Part print with two shaded views. Sizes in mm from the minimum x, y, z corner. Round coordinates to 2 decimals unless told otherwise and drop trailing zeros. Loops run counter-clockwise (first coordinate to the right, second up) from the corner with the lowest first, then second, coordinate; pieces in that order, holes last.
(1) Cut at A-A on z = 0.8. List the corners of the cut face in (x, y) (1 decimal).
(2) Cut at B-B on x = 2. List the corners of the cut face in (y, z).
(3) Cut at D-D on y = 14.5. List the corners of the cut face in (x, z).
(4) Flat gauge pin, fed straight in: pin 1 (5 mm diameter, centred on x = 8, y = 10, fed in from +Z). Where does the tip first touch, or does it go through?
(5) Probe probe 1 along Y at (x, z) = (15, 0.1); probe 2 along Y at (x, z) = (2, 0.3); probe 3 along Z at (x, y) = (1.25, 25.25). List the from-to ranges inside material, lowest first.
(6) Cut at C-C on y = 25. List the corners of the cut face in (x, z).
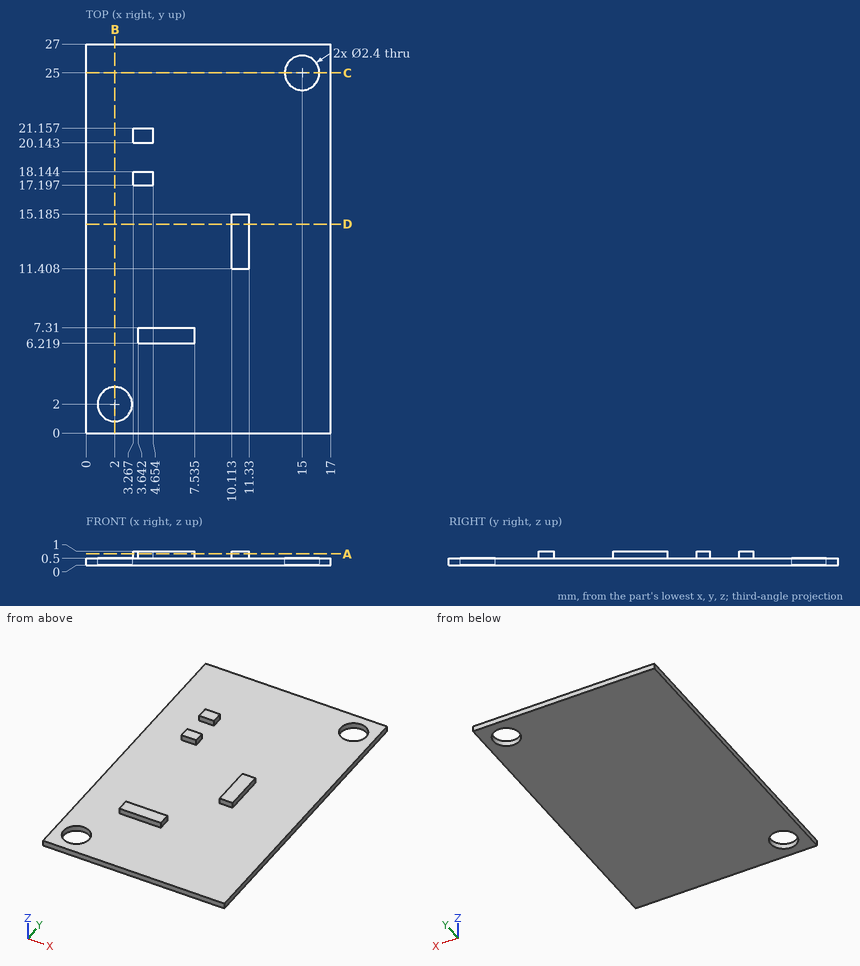
Final values:
1. outline: (3.3, 17.2) - (4.7, 17.2) - (4.7, 18.1) - (3.3, 18.1) - close; (3.3, 20.1) - (4.7, 20.1) - (4.7, 21.2) - (3.3, 21.2) - close; (3.6, 6.2) - (7.5, 6.2) - (7.5, 7.3) - (3.6, 7.3) - close; (10.1, 11.4) - (11.3, 11.4) - (11.3, 15.2) - (10.1, 15.2) - close
2. outline: (0, 0) - (0.8, 0) - (0.8, 0.5) - (0, 0.5) - close; (3.2, 0) - (27, 0) - (27, 0.5) - (3.2, 0.5) - close
3. outline: (0, 0) - (17, 0) - (17, 0.5) - (11.33, 0.5) - (11.33, 1) - (10.11, 1) - (10.11, 0.5) - (0, 0.5) - close
4. pin 1: stops at z = 0.5
5. probe 1: y = 0 to 23.8, 26.2 to 27
5. probe 2: y = 0 to 0.8, 3.2 to 27
5. probe 3: z = 0 to 0.5
6. outline: (0, 0) - (13.8, 0) - (13.8, 0.5) - (0, 0.5) - close; (16.2, 0) - (17, 0) - (17, 0.5) - (16.2, 0.5) - close
